Part model, mm, in its own coordinate system. A direction names the side the tool comes from. Round coordinates to 2 decimals unless told otherwise and drop trailing zeros. Order: outer loops, then holes, each group sorted by start corner. A loop starts at its lowest first (then second) coordinate and runs counter-clockwise, first axis right, second up. Notation, with made-up numbers: (-19, 54) - (-8, 54) arc R14 cw to (-8, 67) - close; hole circle Ø9 at (-31.75, -32.75). An arc over 180 degrees is marked (long way). Return JSON: item names as keys, results as strings. Group by question number.
Item 1: Saw through at B-B on y = 8. List the corners of the cut face in (x, z), and give its area (3 significant figures).
Item 2: Tool access for faces 4 (the face through (50.8, 0, 3)), 5 (the face through (-1.653, 12.592, 6.261)), 6 (the face through (-4, 18, 7.62)), 7 (the face through (7, 12, 0)), 8 (the face through (35.56, 16, 6)): list every direction of +Z, -Z, +X, -X, +Y, -Y with a clear straight run to the whole face (end or side of a thin tool).
Item 3: Saw through at A-A on x = 4.5. List the corners of the cut face in (y, z).
Item 4: Drop flat-ended pins along their axis: pin 1 (6.5 mm diameter, centred on y = 3, z = 7.5, fed in from -X); pin 2 (2.5 mm diameter, centred on x = 42.5, y = 0.5, fed in from +Z); pin 3 (1.5 mm diameter, centred on x = 46, y = -1, fed in from -Z). Give the stop position or say it passes through.
Item 5: Saw through at C-C on x = -17.5. List the corners of the cut face in (y, z).
Item 6: Probe probe 1 along X at (y, z) = (-16, 9); probe 2 along Y at (x, z) = (0, 3.5); probe 3 along Z at (x, y) = (39.5, 0.5). List the from-to ranges inside material, lowest first.
Item 7: Two-plate mould, pull along Y, no slides. Class faces 1 (the face through (45, 0, 8.89)), 2 (the face through (44.36, -1.03, 1.7)), 3 (the face through (4, 18, 7.62)): released by +Y, released by -Y, zero draft, split by the parting line, or undercut.
```python
from build123d import *

# Parameters (mm, degrees)
F0_W      = 76.2
F0_H      = 50.8
F0_R      = 12.7
F1_DEPTH  = 12.7
F2_W      = 1.27
F2_H      = 50.8
F3_DEPTH  = 5.08
F5_DEPTH  = 50.801
F6_R      = 4.7625
F7_DEPTH  = 12.7
F8_W      = 5.08
F8_H      = 50.8
F9_DEPTH  = 5.08
F10_W     = 5.08
F10_H     = 5.08
F11_DEPTH = 12.7
F13_DEPTH = 50.8
F14_R     = 3.175
F15_DEPTH = 2.54
F17_DEPTH = 50.801


# Not quite as in the source:
# - a pattern or mirror of a feature is missing from the dataset's text; its kind, count and spacing are read off the source's solid


with BuildPart() as f1:
    # F0 (on Top) → F1 (new body)
    with BuildSketch(Plane.XY):
        Rectangle(F0_W, F0_H)
        Circle(F0_R, mode=Mode.SUBTRACT)
    extrude(amount=F1_DEPTH)

    # F2 (on face) → F3 (cut)
    with BuildSketch(Plane.XY.offset(12.7)):
        with Locations((-27.305, 0)):
            Rectangle(F2_W, F2_H)
        with BuildLine():
            Line((-6.35, -10.9985226281), (-6.35, -25.4))
            Line((-6.35, -25.4), (6.35, -25.4))
            Line((6.35, -25.4), (6.35, -10.9985226281))
            ThreePointArc((6.35, -10.9985226281), (0, -12.7), (-6.35, -10.9985226281))
        make_face()
        with BuildLine():
            Line((6.35, 25.4), (-6.35, 25.4))
            Line((-6.35, 25.4), (-6.35, 10.9985226281))
            ThreePointArc((-6.35, 10.9985226281), (0, 12.7), (6.35, 10.9985226281))
            Line((6.35, 10.9985226281), (6.35, 25.4))
        make_face()
    extrude(amount=-F3_DEPTH, mode=Mode.SUBTRACT)

    # F4 (on face) → F5 (cut, through all)
    with BuildSketch(Plane.XZ.offset(25.4)):
        Polygon((31.75, 12.7), (19.05, 12.7), (16.1170606325, 7.62), (34.6829393675, 7.62), align=None)
    extrude(amount=-F5_DEPTH, mode=Mode.SUBTRACT)

    # F6 (on face) → F7 (join)
    with BuildSketch(Plane.YZ.offset(38.1)):
        with Locations((0, 6.35)):
            Circle(F6_R)
    extrude(amount=F7_DEPTH)

    # F8 (on face) → F9 (join)
    with BuildSketch(Plane(origin=(0, 0, 0), x_dir=(1, 0, 0), z_dir=(0, 0, -1))):
        with Locations((-35.56, 0)):
            Rectangle(F8_W, F8_H)
        with Locations((35.56, 0)):
            Rectangle(F8_W, F8_H)
    extrude(amount=F9_DEPTH)

    # F10 (on face) → F11 (cut)
    with BuildSketch(Plane.YZ.offset(50.8)):
        with Locations((0, 6.35)):
            Rectangle(F10_W, F10_H)
    extrude(amount=-F11_DEPTH, mode=Mode.SUBTRACT)

    # F12 (on face) → F13 (join, through all)
    with BuildSketch(Plane.XZ.offset(25.4)):
        with BuildLine():
            ThreePointArc((38.1, -5.08), (39.8960512242, -4.3360512242), (40.64, -2.54))
            ThreePointArc((40.64, -2.54), (39.8960512242, -0.7439487758), (38.1, 0))
            Line((38.1, 0), (38.1, -5.08))
        make_face()
        with BuildLine():
            Line((38.1, -5.08), (38.1, 0))
            ThreePointArc((38.1, 0), (35.56, -2.54), (38.1, -5.08))
        make_face()
    f13 = extrude(amount=-F13_DEPTH)

    # F13_copies: F13 across plane
    add(f13.mirror(Plane(origin=(0, 0, 0), x_dir=(0, 0, -1), z_dir=(-1, 0, 0))))

    # F14 (on face) → F15 (cut)
    with BuildSketch(Plane.YZ.offset(38.1)):
        with Locations((-15.875, 6.35)):
            Circle(F14_R)
        with Locations((15.875, 6.35)):
            Circle(F14_R)
    extrude(amount=-F15_DEPTH, mode=Mode.SUBTRACT)

    # F16 (on face) → F17 (cut, through all)
    with BuildSketch(Plane.XZ.offset(25.4)):
        Polygon((-1.5875, 7.62), (0, 6.0325), (1.5875, 7.62), align=None)
    extrude(amount=-F17_DEPTH, mode=Mode.SUBTRACT)


solid = f1.part
```
Filled in:
{
 "1": {"outline": "(-38.1, -5.08) - (-33.02, -5.08) - (-33.02, 0) - (-9.86, 0) - (-9.86, 12.7) - (-26.67, 12.7) - (-26.67, 7.62) - (-27.94, 7.62) - (-27.94, 12.7) - (-38.1, 12.7) - (-38.1, 0) arc R2.54 ccw to start; (9.86, 0) - (33.02, 0) - (33.02, -5.08) - (38.1, -5.08) arc R2.54 ccw to (38.1, 0) - (38.1, 12.7) - (31.75, 12.7) - (34.68, 7.62) - (16.12, 7.62) - (19.05, 12.7) - (9.86, 12.7) - close", "area": "703 mm^2"},
 "2": {"face 4": "+Z, -Z, +X, +Y, -Y", "face 5": "+Z, -Z", "face 6": "+Z, +Y, -Y", "face 7": "-Z, +Y, -Y", "face 8": "+X"},
 "3": {"outline": "(-25.4, 0) - (-11.88, 0) - (-11.88, 7.62) - (-25.4, 7.62) - close; (11.88, 0) - (25.4, 0) - (25.4, 7.62) - (11.88, 7.62) - close"},
 "4": {"pin 1": "stops at x = -38.1", "pin 2": "stops at z = 11.11", "pin 3": "stops at z = 1.59"},
 "5": {"outline": "(-25.4, 0) - (25.4, 0) - (25.4, 12.7) - (-25.4, 12.7) - close"},
 "6": {"probe 1": "x = -38.1 to -27.94, -26.67 to -6.35, 6.35 to 16.91, 33.89 to 35.56", "probe 2": "y = -25.4 to -12.7, 12.7 to 25.4", "probe 3": "z = -4.66 to -0.42, 1.61 to 3.81, 8.89 to 11.09"},
 "7": {"face 1": "undercut", "face 2": "split by the parting line", "face 3": "zero draft"}
}
